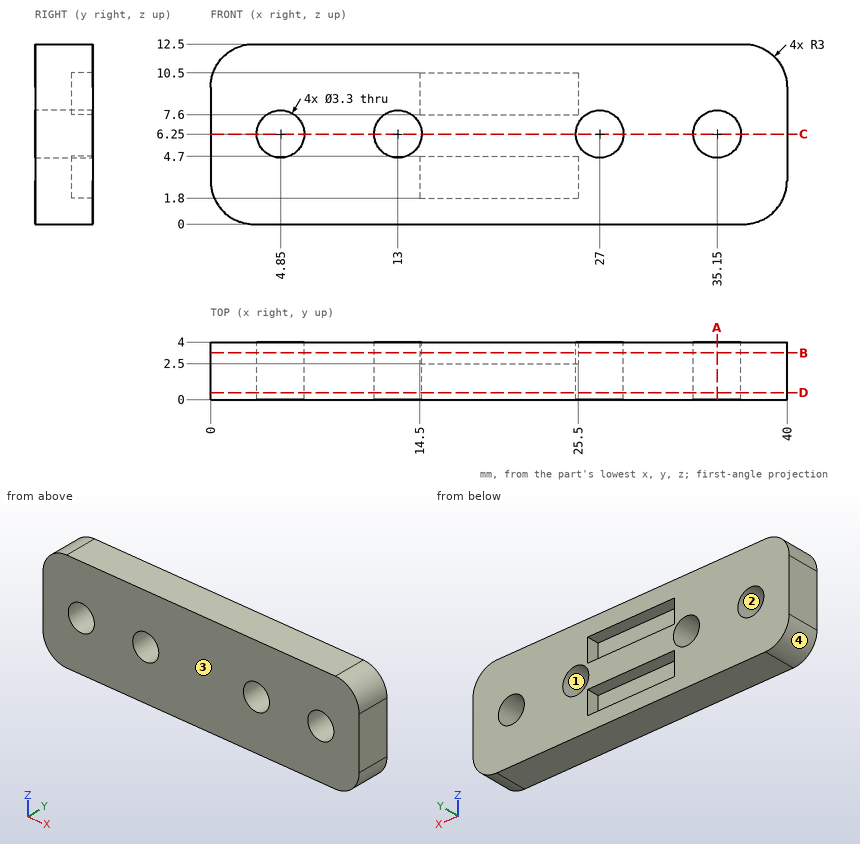
For this review, use the dimensioned drawing (mm, ordinates from the lowest corner) and the shaded views. Coordinates: 2 decimals unless noted, no trailing zeros. Order: outer loops, then holes, each group sorted by start corner. A loop starts at its lowest first (then second) coordinate and runs counter-clockwise, first axis right, second up. Notation, with made-up numbers: M 26.5,-1.5 L 31.5,-1.5 A17 ccw 31.5,2.5 Z; hole C 4,72 d1. An arc over 180 degrees is marked long. Answer as a JSON object with one key per item and string values. Group by question number.
1) For pin 1 (1 mm diameter, centred on y = 1.5, z = 2, fed in from +X), flat-tipped, find the tip position at first contact; note if it passes through.
2) Add section A-A, the plane x = 35.15. Write out the cut boundary in (y, z).
3) Wall thickness on L1, parallel to X at y = 2.35, z = 6.25; L2, parallel to X at y = 1.45, z = 5.25; L3, parallel to X at y = 3.3, z = 9.25: over which ranges is each line inside the solid? List them lowest first.
4) Mouldability with a two-part tool opening along X and no side actions: class the marked faces 1, 2, 3 and 4 as pulls with the +X half, pulls with the -X half, needs draft (parallel to the pull), parting line crosses it, or undercut.
5) Add section B-B, the plane y = 3.25. Write out the cut boundary in (x, z), then the cut area to 3 significant figures.
6) Add section C-C, the plane z = 6.25. Write out the cut boundary in (x, y).
7) Add section D-D, the plane y = 0.5. Write out the cut boundary in (x, z), then the cut area to 3 significant figures.
Computed values:
{
 "1": {"pin 1": "stops at x = 39.96"},
 "2": {"outline": "M 0,0 L 4,0 L 4,4.6 L 0,4.6 Z; M 0,7.9 L 4,7.9 L 4,12.5 L 0,12.5 Z"},
 "3": {"L1": "x = 0 to 3.2, 6.5 to 11.35, 14.65 to 25.35, 28.65 to 33.5, 36.8 to 40", "L2": "x = 0 to 3.54, 6.16 to 11.69, 14.31 to 25.69, 28.31 to 33.84, 36.46 to 40", "L3": "x = 0 to 14.5, 25.5 to 40"},
 "4": {"face 1": "undercut", "face 2": "undercut", "face 3": "needs draft", "face 4": "pulls with the -X half"},
 "5": {"outline": "M 0,3 A3 ccw 3,0 L 37,0 A3 ccw 40,3 L 40,9.5 A3 ccw 37,12.5 L 3,12.5 A3 ccw 0,9.5 Z; hole C 4.85,6.25 d3.3; hole C 13,6.25 d3.3; hole M 14.5,1.8 L 25.5,1.8 L 25.5,4.7 L 14.5,4.7 Z; hole M 14.5,7.6 L 25.5,7.6 L 25.5,10.5 L 14.5,10.5 Z; hole C 27,6.25 d3.3; hole C 35.15,6.25 d3.3", "area": "394 mm^2"},
 "6": {"outline": "M 0,0 L 3.2,0 L 3.2,4 L 0,4 Z; M 6.5,0 L 11.35,0 L 11.35,4 L 6.5,4 Z; M 14.65,0 L 25.35,0 L 25.35,4 L 14.65,4 Z; M 28.65,0 L 33.5,0 L 33.5,4 L 28.65,4 Z; M 36.8,0 L 40,0 L 40,4 L 36.8,4 Z"},
 "7": {"outline": "M 0,3 A3 ccw 3,0 L 37,0 A3 ccw 40,3 L 40,9.5 A3 ccw 37,12.5 L 3,12.5 A3 ccw 0,9.5 Z; hole C 4.85,6.25 d3.3; hole C 13,6.25 d3.3; hole C 27,6.25 d3.3; hole C 35.15,6.25 d3.3", "area": "458 mm^2"}
}
